Geometry: final body of the model. Coordinates: model frame, mm. A direction names the side the tool comes from. Round coordinates to 2 decimals unless told otherwise and drop trailing zeros. Loops run counter-clockwise (first coordinate to the right, second up) from the corner with the lowest first, then second, coordinate; pieces in that order, holes last. Notation, with made-up numbers: M 29.5,46.25 L 80.5,46.25 A10 cw 80.5,54.25 Z; hole C 49,62 d5. An arc over 180 degrees is marked long. Answer as a JSON object with one key per item and string values.
from build123d import *

# Parameters (mm, degrees)
SKETCH1_R  = 1
BODY_DEPTH = 1.2
FILLET1_R  = 4.5


with BuildPart() as part:
    # Sketch1 → Body (new body)
    with BuildSketch(Plane.XY):
        with BuildLine():
            Line((-1.25, -16.329677416), (-1.25, -11.859392549))
            ThreePointArc((-1.25, -11.859392549), (0, 10.27), (1.25, -11.859392549))
            Line((1.25, -11.859392549), (1.25, -16.329677416))
            ThreePointArc((1.25, -16.329677416), (4.338456847, -15.762524642), (7.25, -14.586453031))
            Line((7.25, -14.586453031), (7.25, -11.506411256))
            ThreePointArc((7.25, -11.506411256), (0, 13.6), (-7.25, -11.506411256))
            Line((-7.25, -11.506411256), (-7.25, -14.586453031))
            ThreePointArc((-7.25, -14.586453031), (-4.338456847, -15.762524642), (-1.25, -16.329677416))
        make_face()
        with Locations((-4.25, -13.432678287)):
            Circle(SKETCH1_R, mode=Mode.SUBTRACT)
        with Locations(Location((4.25, -13.432678287, 0), (0, 0, 180))):
            Circle(SKETCH1_R, mode=Mode.SUBTRACT)
    extrude(amount=-BODY_DEPTH)

    # Fillet1
    fillet1_edges = [part.edges().sort_by_distance(p)[0] for p in [
        (7.25, -11.506411256, -0.6),
        (-7.25, -11.506411256, -0.6),
    ]]
    fillet(fillet1_edges, radius=FILLET1_R)


solid = part.part
1) Section query A-A (y = -9.75). Return the cut outline in (x, z).
Results:
{"outline": "M -9.48,-1.2 L -6.61,-1.2 L -6.61,0 L -9.48,0 Z; M 6.61,-1.2 L 9.48,-1.2 L 9.48,0 L 6.61,0 Z"}
2) Reachability of faces 1 (the flat face through (1.25, -14, -1)), 2 (the flat face through (-7.25, -14, -1)), 3 (the flat face through (-11.14, 0.92, -1.2)) from +Z, -Z, +X, -X, +Y, -Y: full face, straight path, thin tool, end or side. Return the list, or none.
Results:
{"face 1": "+Z, -Z, -Y", "face 2": "+Z, -Z, -X, -Y", "face 3": "-Z, +X, -X, +Y, -Y"}
3) Pull-direction query (Y, two-part tool) for faces 4 (the flat face through (7.25, -14, -1)), 5 (the cylindrical face through (-4.99, -12.76, -0.59)), 6 (the cylindrical face through (-4.38, -15.75, -0.59)); classes: +Y half, -Y half, draft (parallel to the pull), parting line (faces both ways), or undercut.
Results:
{"face 4": "draft", "face 5": "undercut", "face 6": "-Y half"}
4) Ray query, line 1 (Y direction, x = -4.5, z = -0.25); line 2 (X direction, y = -4.5, z = -0.25); line 3 (Y direction, x = 9.75, z = -0.25). Return the intervals inside material, ascending.
Results:
{"line 1": "-15.71 to -14.4, -12.46 to -10.98, 9.32 to 12.83", "line 2": "-12.83 to -10.48, 10.48 to 12.83", "line 3": "-9.48 to -6.14, 4.48 to 9.48"}
5) Section query C-C (z = -0.55). Return the cut outline in (x, y).
Results:
{"outline": "M -8.83,-10.34 A4.5 cw -7.25,-13.77 L -7.25,-14.59 A15.55 ccw -1.25,-16.33 L -1.25,-11.86 A11.1 cw long 1.25,-11.86 L 1.25,-16.33 A15.55 ccw 7.25,-14.59 L 7.25,-13.77 A4.5 cw 8.83,-10.34 A13.6 ccw long Z; hole C -4.25,-13.43 d2; hole C 4.25,-13.43 d2"}
6) Section query B-B (x = 4.25). Return the cut outline in (y, z).
Results:
{"outline": "M -15.79,-1.2 L -14.43,-1.2 L -14.43,0 L -15.79,0 Z; M -12.43,-1.2 L -11.08,-1.2 L -11.08,0 L -12.43,0 Z; M 9.42,-1.2 L 12.92,-1.2 L 12.92,0 L 9.42,0 Z"}
7) Section query D-D (x = -8). Return the cut outline in (y, z), and give its area (3 significant figures).
Results:
{"outline": "M -11.28,-1.2 L -8.52,-1.2 L -8.52,0 L -11.28,0 Z; M 6.86,-1.2 L 11,-1.2 L 11,0 L 6.86,0 Z", "area": "8.27 mm2"}
8) Pin query (flat end, axial travel): P1, Ø0.6, axis at y = -14.5, z = -0.5, coming from the -X side. Return the tip coordinate at first contact, or that it passes through.
Results:
{"P1": "x = -7.25"}
